from build123d import *

# Parameters (mm, degrees)
F1_DEPTH = 3
F2_DEPTH = 5
F3_DEPTH = 10
F5_DEPTH = 1
F6_DEPTH = 2


with BuildPart() as f1:
    # F0 (on Top) → F1 (new body)
    with BuildSketch(Plane.XY):
        Polygon((15, -15), (-15, -15), (-15, 12.604296), (-15, 18), (-70, 18), (-70, -82), (70, -82), (70, 18), (15, 18), (15, 12.604296), align=None)
        Polygon((-2.5, -77), (-65, -77), (-65, 13), (-20, 13), (-20, -20), (-2.5, -20), align=None, mode=Mode.SUBTRACT)
        Polygon((2.5, -20), (20, -20), (20, 13), (65, 13), (65, -77), (2.5, -77), align=None, mode=Mode.SUBTRACT)
        Polygon((-15, 12.604296), (-15, -15), (15, -15), (15, 12.604296), (12, 12.604296), (12, 18), (-12, 18), (-12, 12.604296), align=None)
        with BuildLine():
            ThreePointArc((4, 9.165151), (8.3666, 5.477226), (10, 0))
            ThreePointArc((10, 0), (-5.477226, -8.3666), (-4, 9.165151))
            Line((-4, 9.165151), (-4, 15))
            Line((-4, 15), (4, 15))
            Line((4, 15), (4, 9.165151))
        make_face(mode=Mode.SUBTRACT)
    extrude(amount=F1_DEPTH)

    # F0 (on Top) → F2 (join)
    with BuildSketch(Plane.XY):
        Polygon((-15, 12.604296), (-15, -15), (15, -15), (15, 12.604296), (12, 12.604296), (12, 18), (-12, 18), (-12, 12.604296), align=None)
        with BuildLine():
            ThreePointArc((4, 9.165151), (8.3666, 5.477226), (10, 0))
            ThreePointArc((10, 0), (-5.477226, -8.3666), (-4, 9.165151))
            Line((-4, 9.165151), (-4, 15))
            Line((-4, 15), (4, 15))
            Line((4, 15), (4, 9.165151))
        make_face(mode=Mode.SUBTRACT)
    extrude(amount=F2_DEPTH)

    # F0 (on Top) → F3 (join)
    with BuildSketch(Plane.XY):
        with BuildLine():
            ThreePointArc((-4, 9.165151), (0, 10), (4, 9.165151))
            Line((4, 9.165151), (4, 15))
            Line((4, 15), (-4, 15))
            Line((-4, 15), (-4, 9.165151))
        make_face()
        with BuildLine():
            Line((4, 0), (4, 9.165151))
            ThreePointArc((4, 9.165151), (0, 10), (-4, 9.165151))
            Line((-4, 9.165151), (-4, 0))
            Line((-4, 0), (4, 0))
        make_face()
        with BuildLine():
            ThreePointArc((-4, 9.165151), (-5.477226, -8.3666), (10, 0))
            ThreePointArc((10, 0), (8.3666, 5.477226), (4, 9.165151))
            Line((4, 9.165151), (4, 0))
            Line((4, 0), (-4, 0))
            Line((-4, 0), (-4, 9.165151))
        make_face()
    extrude(amount=F3_DEPTH)

    # F4 (on Right) → F5 (join, symmetric)
    with BuildSketch(Plane.YZ):
        Polygon((-15, 3), (-15, 5), (-48.5, 3), align=None)
    extrude(amount=F5_DEPTH, both=True)

    # F0 (on Top) → F6 (join)
    with BuildSketch(Plane.XY):
        Polygon((-65, 13), (-65, -77), (-2.5, -77), (-2.5, -20), (-20, -20), (-20, 13), align=None)
        Polygon((20, 13), (20, -20), (2.5, -20), (2.5, -77), (65, -77), (65, 13), align=None)
    extrude(amount=F6_DEPTH)


solid = f1.part
Read the model definition and answer for the solid it produces. Units are mm, in the model's axes. A direction names the side the tool comes from. Round coordinates to 2 decimals unless told otherwise and drop trailing zeros. Order: outer loops, then holes, each group sorted by start corner. A loop starts at its lowest first (then second) coordinate and runs counter-clockwise, first axis right, second up.
1) For faces 1 (the face through (-42, 18, 1)), 2 (the face through (-4, 12, 7)), 3 (the face through (-15, 15, 1)), 4 (the face through (-1, -31, 0)), 5 (the face through (0, 15, 7)), determine the directions among +Z, -Z, +X, -X, +Y, -Y from which every point of the face is accessible in a straight line to the end or side of a thin tool.
2) The part is cut by section C-C on y = -12. Write down the section's boundary in (x, z).
3) Flat-ended cylindrical pins translate along their axes: pin 1 (1.5 mm diameter, centred on x = 13, z = 2, fed in from +Y); pin 2 (1 mm diameter, centred on y = 1, z = 6.5, fed in from +X); pin 3 (1 mm diameter, centred on y = -31.5, z = 4, fed in from +X); pin 4 (1.5 mm diameter, centred on x = -43, z = 5.5, fed in from +Y). Find the tip coordinate at first contact, or state that the pin passes through.
4) The mould has two halves that part along X. Classify faces 6 (the face through (4, 12, 7)), 7 (the face through (-13, 12.604, 2)), 8 (the face through (5, -17, 3)): released by +X, released by -X, zero draft, split by the parting line, or undercut.
5) The part is cut by section A-A on y = -68. Write down the section's boundary in (x, z).
6) The part is cut by section B-B on x = -52.5. Write down the section's boundary in (y, z), plus the area to 3 significant figures.
7) Straight lines are drawn through the part: L1, parallel to X at y = -60, z = 2.75; L2, parallel to X at y = -6.5, z = 2.5; L3, parallel to Z at x = 15.5, y = -28.5. For each, find the intervals that lie inside material, in ascending order.
8) The part is cut by section D-D on y = -43. Write down the section's boundary in (x, z).
Resolved:
1. face 1: +Z, -Z, +X, -X, +Y
1. face 2: +Z, -X, +Y
1. face 3: +Z, -Z, +Y
1. face 4: -Z, +X, -X, +Y, -Y
1. face 5: +Z, +X, -X, +Y
2. outline: (-70, 0) - (70, 0) - (70, 3) - (65, 3) - (65, 2) - (20, 2) - (20, 3) - (15, 3) - (15, 5) - (-15, 5) - (-15, 3) - (-20, 3) - (-20, 2) - (-65, 2) - (-65, 3) - (-70, 3) - close
3. pin 1: stops at y = 12.6
3. pin 2: stops at x = 9.99
3. pin 3: stops at x = 1
3. pin 4: passes through
4. face 6: released by +X
4. face 7: undercut
4. face 8: zero draft
5. outline: (-70, 0) - (70, 0) - (70, 3) - (65, 3) - (65, 2) - (2.5, 2) - (2.5, 3) - (-2.5, 3) - (-2.5, 2) - (-65, 2) - (-65, 3) - (-70, 3) - close
6. outline: (-82, 0) - (18, 0) - (18, 3) - (13, 3) - (13, 2) - (-77, 2) - (-77, 3) - (-82, 3) - close
6. area: 210 mm2
7. L1: x = -70 to -65, -2.5 to 2.5, 65 to 70
7. L2: x = -70 to -65, -20 to 20, 65 to 70
7. L3: z = 0 to 2
8. outline: (-70, 0) - (70, 0) - (70, 3) - (65, 3) - (65, 2) - (2.5, 2) - (2.5, 3) - (1, 3) - (1, 3.33) - (-1, 3.33) - (-1, 3) - (-2.5, 3) - (-2.5, 2) - (-65, 2) - (-65, 3) - (-70, 3) - close
